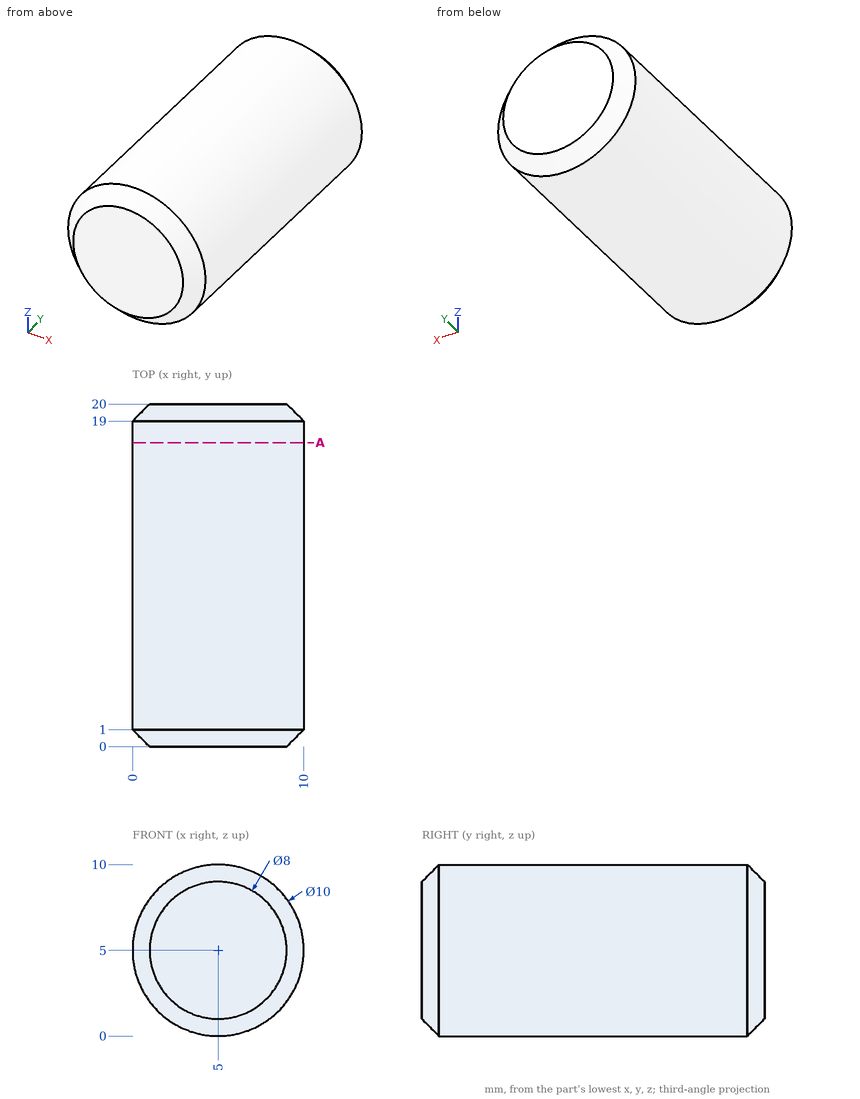
Check sheet for the drawn part. Datum: minimum x, y, z corner. Units: mm. Round coordinates to 2 decimals unless told otherwise and drop trailing zeros. Order: outer loops, then holes, each group sorted by start corner. A loop starts at its lowest first (then second) coordinate and runs counter-clockwise, first axis right, second up. Notation, with made-up numbers: M 72.25,8.5 L 88.25,8.5 A34 cw 88.25,42.5 Z; hole C -37,59 d6. An arc over 180 degrees is marked long. Answer in a Markdown table with one row per item.
(1) Section check A-A on y = 17.75. Record the boundary of the cut face in (x, z).
Findings:
| item | result |
|---|---|
| outline | C 5,5 d10 |
(2) Gauge pin test, flat ends, axial feed: pin 1 (1 mm diameter, centred on x = 6.5, y = 9, fed in from +Z); pin 2 (1 mm diameter, centred on y = 14, z = 8.5, fed in from -X). Record the tip position at first contact, or that the pin passes through.
Findings:
| item | result |
|---|---|
| pin 1 | stops at z = 9.9 |
| pin 2 | stops at x = 1 |
(3) Material ranges on line 1 along X through (y, z) = (8.75, 2); line 2 along Z through (x, y) = (8.75, 11.75), recorded low to high. Write a range as from..to.
Findings:
| item | result |
|---|---|
| line 1 | x = 1..9 |
| line 2 | z = 1.69..8.31 |
